Input: part model. Units: mm. Frame: model coordinates. Face numbers are marked on the shaded views. A direction names the side the tool comes from. Give positions to 0.01 mm unless a question says otherwise; leave off trailing zeros. Write each loop counter-clockwise with the first axis right and the second up, starting at its lowest first coordinate (ties: lowest second). Pieces come first, ordered by that corner, then holes. Notation, with made-up numbers: M -11,-8.5 L 12,-8.5 A23 ccw 12,14.5 Z; hole C 39.5,34 d4. An arc over 180 degrees is marked long. Use CSV: the item, a comma, the result in double quotes. Start each with the question number.
from build123d import *

# Parameters (mm, degrees)
MAINBODYS_W                           = 6.4
MAINBODYS_H                           = 0.8
MAIN_BODY_DEPTH                       = 12
BOTTOM_OF_MAIN_BODY_REACH             = 14.426
BOTTOM_OF_MAIN_BODY_DIRECTION_2_REACH = 14.426
TOPHOLES_R                            = 0.9
TOP_HOLE_DEPTH                        = 13.840950121
F_45_DEGREE_FLANGE_DEPTH              = 2
BOTTOM_FLAT_FLANGE_DEPTH              = 2
EXTENDEDBOTTOMFLANGES_W               = 3
EXTENDEDBOTTOMFLANGES_H               = 0.8
EXTENDED_BOTTOM_FLANGE_DEPTH          = 0.8
BOSSEDCYLINDERBODYS_R                 = 1.45
BOSSED_CYLINDER_BODY_DEPTH            = 0.8
C_MAIN_BODY_SIZE                      = 1


# Sheet-metal steps are written as plain solids
with BuildPart() as part:
    # MainBodyS → MAIN BODY (new body)
    with BuildSketch(Plane(origin=(0, 0, 0), x_dir=(1, 0, 0), z_dir=(0, 1, 0))):
        Rectangle(MAINBODYS_W, MAINBODYS_H)
    extrude(amount=MAIN_BODY_DEPTH)

    # BOTTOM OF MAIN BODY: up to this face of the body (flat: up to its plane)
    bottom_of_main_body_end = Plane(part.part.faces().sort_by_distance((0, 6, 0.4))[0])
    # BottomMainBodyS → BOTTOM OF MAIN BODY (add, up to the picked face)
    with BuildSketch(Plane.XY, mode=Mode.PRIVATE) as bottom_of_main_body_sk1:
        Polygon((0, 0), (4, 0), (4, -2), (4.5, -5), (2.9, -5), (1.5, -2.2), (0, -2.2), align=None)
    bottom_of_main_body_tool1 = split(extrude(bottom_of_main_body_sk1.sketch, amount=BOTTOM_OF_MAIN_BODY_REACH, mode=Mode.PRIVATE), bisect_by=bottom_of_main_body_end, keep=Keep.BOTH, mode=Mode.PRIVATE)
    bottom_of_main_body = bottom_of_main_body_tool1.solids().sort_by(Axis((2.475691, -2.049989, 0), (0, 0, 1)))[0]
    add(bottom_of_main_body)

    # BOTTOM OF MAIN BODY direction 2: up to this face of the body (flat: up to its plane)
    bottom_of_main_body_direction_2_end = Plane(part.part.faces().sort_by_distance((0, 6, -0.4))[0])
    # BottomMainBodyS → BOTTOM OF MAIN BODY direction 2 (add, up to the picked face)
    with BuildSketch(Plane.XY, mode=Mode.PRIVATE) as bottom_of_main_body_direction_2_sk1:
        Polygon((0, 0), (4, 0), (4, -2), (4.5, -5), (2.9, -5), (1.5, -2.2), (0, -2.2), align=None)
    bottom_of_main_body_direction_2_tool1 = split(extrude(bottom_of_main_body_direction_2_sk1.sketch, amount=-BOTTOM_OF_MAIN_BODY_DIRECTION_2_REACH, mode=Mode.PRIVATE), bisect_by=bottom_of_main_body_direction_2_end, keep=Keep.BOTH, mode=Mode.PRIVATE)
    bottom_of_main_body_direction_2 = bottom_of_main_body_direction_2_tool1.solids().sort_by(Axis((2.475691, -2.049989, 0), (0, 0, -1)))[0]
    add(bottom_of_main_body_direction_2)

    # BMB HM: BOTTOM OF MAIN BODY, BOTTOM OF MAIN BODY direction 2 across plane
    add(bottom_of_main_body.mirror(Plane(origin=(0, 0, 0), x_dir=(0, 0, 1), z_dir=(1, 0, 0))))
    add(bottom_of_main_body_direction_2.mirror(Plane(origin=(0, 0, 0), x_dir=(0, 0, 1), z_dir=(1, 0, 0))))

    # TopHoleS → TOP HOLE (cut, through all)
    with BuildSketch(Plane.XY.offset(0.4)):
        with Locations((0, 7)):
            Circle(TOPHOLES_R)
    extrude(amount=-TOP_HOLE_DEPTH, mode=Mode.SUBTRACT)

    # 45 DEGREE FLANGE section (across the edge) → 45 DEGREE FLANGE (add)
    with BuildSketch(Plane(origin=(1, -2.365685425, -0.4), x_dir=(0, 0.7071067811865438, -0.7071067811865512), z_dir=(-1, 0, 0))):
        with BuildLine():
            Line((-0.8, 0.165685425), (-0.8, 2.2))
            Line((-0.8, 2.2), (0, 2.2))
            Line((0, 2.2), (0, 0.165685425))
            ThreePointArc((0, 0.165685425), (0.030448187, 0.012612052), (0.117157288, -0.117157288))
            Line((0.117157288, -0.117157288), (-0.448528137, -0.682842712))
            ThreePointArc((-0.448528137, -0.682842712), (-0.708655439, -0.293534694), (-0.8, 0.165685425))
        make_face()
    extrude(amount=F_45_DEGREE_FLANGE_DEPTH)

    # BOTTOM FLAT FLANGE section (across the edge) → BOTTOM FLAT FLANGE (add)
    with BuildSketch(Plane(origin=(-1, -5.169848481, -2.072792206), x_dir=(0, 1, 0), z_dir=(1, 0, 0))):
        with BuildLine():
            Line((-0.8, 0.965685425), (-0.8, 1.5))
            Line((-0.8, 1.5), (0, 1.5))
            Line((0, 1.5), (0, 0.965685425))
            ThreePointArc((0, 0.965685425), (0.246926627, 0.596133612), (0.682842712, 0.682842712))
            Line((0.682842712, 0.682842712), (1.248528137, 0.117157288))
            ThreePointArc((1.248528137, 0.117157288), (-0.059220119, -0.142970014), (-0.8, 0.965685425))
        make_face()
    extrude(amount=BOTTOM_FLAT_FLANGE_DEPTH)

    # ExtendedBottomFlangeS → EXTENDED BOTTOM FLANGE (add)
    with BuildSketch(Plane.XY.offset(-0.572792206)):
        with Locations((0, -5.569848481)):
            Rectangle(EXTENDEDBOTTOMFLANGES_W, EXTENDEDBOTTOMFLANGES_H)
    extrude(amount=EXTENDED_BOTTOM_FLANGE_DEPTH)

    # BossedCylinderBodyS → BOSSED  CYLINDER BODY (add)
    with BuildSketch(Plane.XZ.offset(5.969848481)):
        with BuildLine():
            Line((-1.5, 0.227207794), (1.5, 0.227207794))
            ThreePointArc((1.5, 0.227207794), (0, 4.614344857), (-1.5, 0.227207794))
        make_face()
        with Locations(Location((0, 2.164344857, 0), (0, 0, 270))):
            Circle(BOSSEDCYLINDERBODYS_R, mode=Mode.SUBTRACT)
    extrude(amount=-BOSSED_CYLINDER_BODY_DEPTH)

    # C MAIN BODY
    c_main_body_edges = [part.edges().sort_by_distance(p)[0] for p in [
        (-3.2, 12, 0),
        (3.2, 12, 0),
    ]]
    chamfer(c_main_body_edges, length=C_MAIN_BODY_SIZE)


solid = part.part
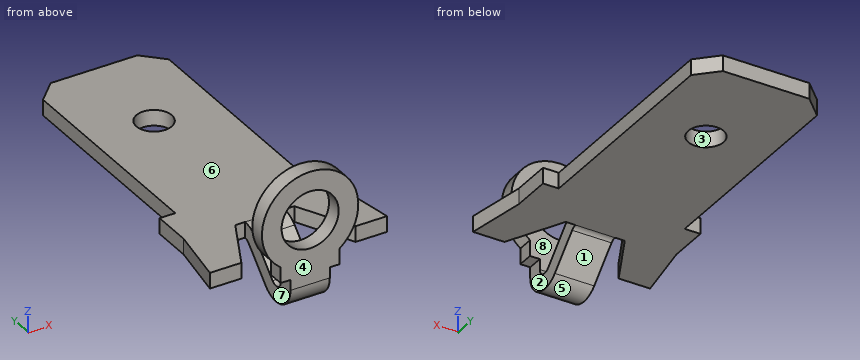
Q1. Section C-C, the plane z = 2.25. Return the cut outline in (x, y), and give its area (3 significant figures).
Q2. Pull-direction query (X, two-part tool) for the marked faces 1, 2 and 3; classes: released by +X, released by -X, zero draft, split by the parting line, or undercut.
Q3. Section B-B, the plane y = 7. Return the cut outline in (x, z).
Q4. Material intervals for L1, parallel to Y at x = 0, z = 0.15; L2, parallel to Y at x = 0, z = 0.1; L3, parallel to Z at x = -3, y = 0, sorted ascending. Write a range as [from, to].
Q5. Section A-A, the plane x = 0. Return the cut outline in (y, z).
Q6. Section D-D, the plane y = -2.75. Return the cut outline in (x, z) (3 decimals), and give its area (3 significant figures).
Q7. Set-up query: the marked faces 4, 5, 6, 7 and 8. Return all of +Z, -Z, +X, -X, +Y, -Y with unobstructed straight access to the full face (end or side cutting, diameter ignored); none if empty.
Q8. First-contact query: pin 1 Ø4 at (x, z) = (-0.5, 2.5) entering from +Y; pin 2 Ø1.4 at (y, z) = (-5, -1.5) entering from +X; pin 3 Ø2 at (x, y) = (0, 7) entering from -Z. Flat tips, straight axial feed; report the tip coordinate or a pass-through.
Check result:
1,outline,"M -2.45,-5.97 L -1.45,-5.97 L -1.45,-5.17 L -2.45,-5.17 Z; M 1.45,-5.97 L 2.45,-5.97 L 2.45,-5.17 L 1.45,-5.17 Z"
1,area,"1.60 mm²"
2,face 1,"zero draft"
2,face 2,"undercut"
2,face 3,"undercut"
3,outline,"M -3.2,-0.4 L -0.9,-0.4 L -0.9,0.4 L -3.2,0.4 Z; M 0.9,-0.4 L 3.2,-0.4 L 3.2,0.4 L 0.9,0.4 Z"
4,L1,"y = [-5.97, -5.17], [-2.93, 6.1], [7.9, 12]"
4,L2,"y = [-5.97, -5.17], [-2.99, 6.1], [7.9, 12]"
4,L3,"z = [-0.4, 0.4]"
5,outline,"M -5.97,-1.11 A1.2 ccw -3.92,-1.96 L -2.48,-0.52 A0.4 cw -2.2,-0.4 L 6.1,-0.4 L 6.1,0.4 L -2.2,0.4 A1.2 ccw -3.05,0.05 L -4.49,-1.39 A0.4 cw -5.17,-1.11 L -5.17,0.71 L -5.97,0.71 Z; M -5.97,3.61 L -5.17,3.61 L -5.17,4.61 L -5.97,4.61 Z; M 7.9,-0.4 L 12,-0.4 L 12,0.4 L 7.9,0.4 Z"
6,outline,"M -4.125,-0.4 L -1.775,-0.4 L -1.775,0.4 L -4.125,0.4 Z; M -1,-0.784 L 1,-0.784 L 1,0.267 L -1,0.267 Z; M 1.775,-0.4 L 4.125,-0.4 L 4.125,0.4 L 1.775,0.4 Z"
6,area,"5.86 mm²"
7,face 4,"+Z, -Z, +X, -X, -Y"
7,face 5,"-Z, +X, -X"
7,face 6,"+Z, +X, -X, +Y"
7,face 7,"-Z"
7,face 8,"+Z, +X, -X"
8,pin 1,"stops at y = -5.17"
8,pin 2,"stops at x = 1"
8,pin 3,"stops at z = -0.4"
